Autodesk Inventor part; units mm, degrees
ref_plane "Cross Section Plane" through (1.9319, 18.3368, 0) normal (1, -0.0018, 0) x (0, 0, 1)
ref_plane "Work Plane2" through (1.9231, 13.5622, 0) normal (-1, 0, 0) x (0, 0, 1)
ref_plane "Work Plane3" through (71.0893, 13.5622, 0) normal (0.9951, -0.0987, 0) x (0, 0, 1)
sketch "Sketch Path" plane through (0, 0, 0) normal (0, 0, 1) x (1, 0, 0)
  arc A0 (1.9319, 18.3368) -> (1.9319, 8.7876) centre (1.9231, 13.5622) ccw
  arc A1 (16.2894, 8.7353) -> (15.407, 8.8122) centre (15.4161, 3.8122) ccw
  arc A2 (68.5875, -0.5416) -> (68.5875, 27.666) centre (71.0893, 13.5622) ccw
  arc A3 (15.407, 18.3122) -> (16.2894, 18.3891) centre (15.4161, 23.3122) ccw
  line L0 (15.407, 18.3122) -> (1.9319, 18.3368)
  line L1 (1.9319, 8.7876) -> (15.407, 8.8122)
  line L2 (16.2894, 8.7353) -> (68.5875, -0.5416)
  line L3 (68.5875, 27.666) -> (16.2894, 18.3891)
ref_plane "Cross Section Plane" through (1.9319, 18.3368, 0) normal (1, -0.0018, 0) x (0, 0, 1)
ref_plane "Work Plane2" through (1.9231, 13.5622, 0) normal (-1, 0, 0) x (0, 0, 1)
ref_plane "Work Plane3" through (71.0893, 13.5622, 0) normal (0.9951, -0.0987, 0) x (0, 0, 1)
sketch "Cross Section" plane through (1.9319, 18.3368, 0) normal (1, -0.0018, 0) x (0, 0, 1)
  line L0 (-2, 0.3) -> (2, 0.3)
  line L1 (2, 0.3) -> (2, -0.3)
  line L2 (2, -0.3) -> (-2, -0.3)
  line L3 (-2, -0.3) -> (-2, 0.3)
  line L4 (-2, 0) -> (2, 0) construction
  point P0 (0, 0)
  point P1 (0, 0)
  dimension "d0" = 4
  dimension "d4" = 0.3
  dimension "d5" = 0.3
sweep "Belt" add profiles "Cross Section" path "Sketch Path"
equation "\"d0\" = da_B"
equation "\"d4\" = da_a"
equation "\"d5\" = da_a2"
equation "\"da_B\" = 4"
equation "\"da_pb\" = 2.5"
equation "\"da_a\" = 0.3"
equation "\"da_S\" = 1.5"
equation "\"da_Beta\" = 20deg"
equation "\"da_Ht\" = 0.7"
equation "\"da_H\" = 1.3"
equation "\"da_a2\" = 0.3"
properties part number "Synchronous Belt" material "Rubber"
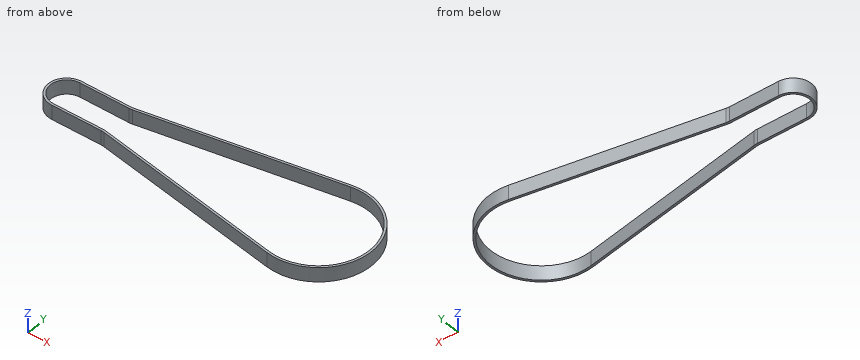
Source: CAD feature listing. Evaluate the final solid. Frame: model axes, mm. Round coordinates to 2 decimals unless told otherwise and drop trailing zeros. Write each loop counter-clockwise with the first axis right and the second up, starting at its lowest first coordinate (ties: lowest second). Pieces come first, ordered by that corner, then holes. Notation, with made-up numbers: M 7.5,-4 L 57.5,-4 A4 cw 57.5,1 Z; hole C -27,-16 d7. An arc over 180 degrees is marked long. One line per item, written item: value. Start each with the question number.
Item 1: Section query C-C (x = 10.5). Return the cut outline in (y, z), plus the area to 3 significant figures.
Item 2: Section query A-A (z = 1.4). Return the cut outline in (x, y).
Item 3: Section query B-B (y = 24). Return the cut outline in (x, z), plus the area to 3 significant figures.
Item 4: Pin query (flat end, axial travel): pin 1 (8 mm diameter, centred on x = 65.5, y = 22, fed in from -Z); pin 2 (1.5 mm diameter, centred on x = 29.5, z = -1.5, fed in from +Y). Return the tip coordinate at first contact, or that it passes through.
Item 5: Ray query, L1, parallel to Y at x = 13.5, z = -0.9; L2, parallel to Y at x = 71, z = 1.3; L3, parallel to X at y = 17.5, z = -0.1. Return the intervals inside material, ascending. Write a range as from..to.
Result set:
1. outline: M 8.5,-2 L 9.1,-2 L 9.1,2 L 8.5,2 Z; M 18.02,-2 L 18.62,-2 L 18.62,2 L 18.02,2 Z
1. area: 4.80 mm²
2. outline: M 1.93,8.49 L 15.41,8.51 A4.71 cw 16.24,8.44 L 68.54,-0.84 A14.62 ccw long 68.54,27.96 L 16.24,18.68 A4.69 cw 15.41,18.61 L 1.93,18.64 A5.07 ccw Z; hole M 1.93,9.09 L 15.41,9.11 A5.31 cw 16.34,9.03 L 68.64,-0.25 A14.02 ccw long 68.64,27.37 L 16.34,18.09 A5.29 cw 15.41,18.01 L 1.93,18.04 A4.47 ccw Z
3. outline: M 46.2,-2 L 49.64,-2 L 49.64,2 L 46.2,2 Z; M 80.46,-2 L 81.33,-2 L 81.33,2 L 80.46,2 Z
3. area: 17.2 mm²
4. pin 1: passes through
4. pin 2: stops at y = 21.17
5. L1: y = 8.51..9.11, 18.02..18.62
5. L2: y = -1.06..-0.46, 27.59..28.19
5. L3: x = -1.28..-0.2, 84.55..85.17
